The figure shows three views and two pictorial views of one solid part (mm, origin at its lowest corner). Answer the questions. Give positions to 0.01 mm unless a question says otherwise; leave off trailing zeros. Order: outer loops, then holes, each group sorted by start corner. A loop starts at its lowest first (then second) coordinate and runs counter-clockwise, first axis right, second up. Notation, with made-up numbers: M 65.25,-29.75 L 88.25,-29.75 A25 ccw 88.25,5.25 Z; hole C -24.5,26 d7. An arc over 180 degrees is marked long. One line per item, written item: value.
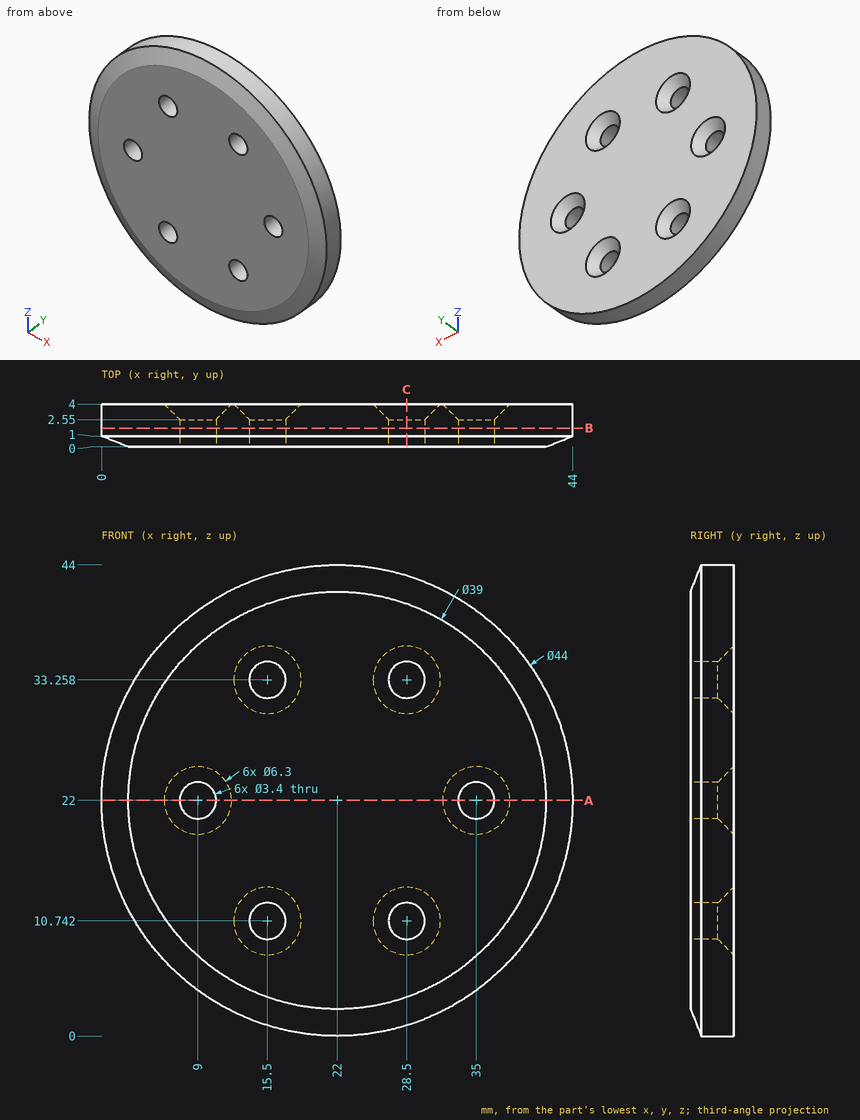
1) Each of these flat-tipped pins is pushed along its axis until it touches: pin 1 Ø10 at (x, z) = (23, 30.5) entering from -Y; pin 2 Ø4 at (x, z) = (9, 22) entering from +Y; pin 3 Ø5.5 at (x, z) = (28.5, 10.74) entering from +Y; pin 4 Ø1.5 at (x, y) = (17.5, 2) entering from -Z. Where does it stop, or does it pass through?
Reported:
pin 1: stops at y = 0
pin 2: stops at y = 2.85
pin 3: stops at y = 3.6
pin 4: stops at z = 0.32
2) Consider probe 1 along X at (y, z) = (0.7, 22); probe 2 along Z at (x, y) = (15.5, 1.85); probe 3 along X at (y, z) = (3.3, 20) (1 decimal). Determine where each line is inside the solid, lowest interval first.
Reported:
probe 1: x = 0.75 to 7.3, 10.7 to 33.3, 36.7 to 43.25
probe 2: z = 0.98 to 9.04, 12.44 to 31.56, 34.96 to 43.02
probe 3: x = 0.1 to 7.6, 10.4 to 33.6, 36.4 to 43.9
3) Find section B-B, the plane y = 1.75. Write down the section's boundary in (x, z), plus the area to 3 significant figures.
Reported:
outline: C 22,22 d44; hole C 9,22 d3.4; hole C 15.5,10.74 d3.4; hole C 15.5,33.26 d3.4; hole C 28.5,10.74 d3.4; hole C 28.5,33.26 d3.4; hole C 35,22 d3.4
area: 1,470 mm^2
4) Find section A-A, the plane z = 22. Write down the section's boundary in (x, y).
Reported:
outline: M 0,1 L 2.5,0 L 7.3,0 L 7.3,2.55 L 5.85,4 L 0,4 Z; M 10.7,0 L 33.3,0 L 33.3,2.55 L 31.85,4 L 12.15,4 L 10.7,2.55 Z; M 36.7,0 L 41.5,0 L 44,1 L 44,4 L 38.15,4 L 36.7,2.55 Z
5) Find section C-C, the plane x = 28.5. Count the separate pieces of the cut face and the enclosed holes in it, plus the area to 3 significant figures.
Reported:
separate pieces: 3
enclosed holes: 0
area: 134 mm^2
